Build history of the part. All positions in model axes, mm. Face numbers are marked on the shaded views. A direction names the side the tool comes from. Coordinates: 2 decimals unless noted, no trailing zeros. Order: outer loops, then holes, each group sorted by start corner. A loop starts at its lowest first (then second) coordinate and runs counter-clockwise, first axis right, second up. Notation, with made-up numbers: (19, 13) -> (77, 13) arc R10 ccw to (77, 26) -> close; hole circle Ø3 at (78.5, 35.5). An arc over 180 degrees is marked (long way). Write each question's results on one line, items separated by ' | '.
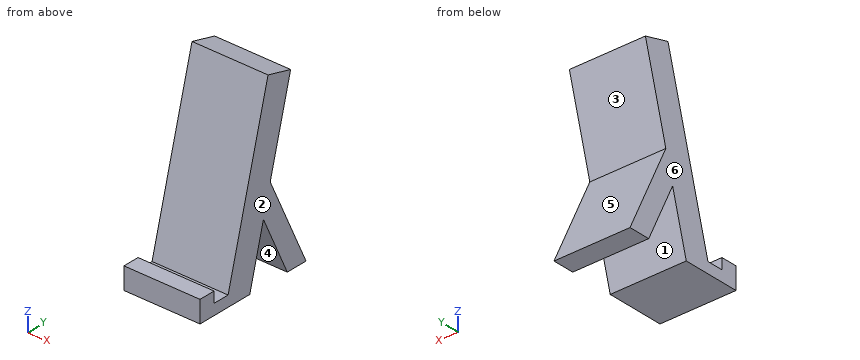
from build123d import *

# Parameters (mm, degrees)
F0_W     = 63.5
F0_H     = 25.4
F1_DEPTH = 19.05
F2_W     = 19.05
F2_H     = 12.7
F3_DEPTH = 63.5
F4_DEPTH = 25.4
F6_DEPTH = 88.9


with BuildPart() as f1:
    # F0 (on Front) → F1 (new body)
    with BuildSketch(Plane.XZ):
        with Locations((-31.75, 12.7)):
            Rectangle(F0_W, F0_H)
    extrude(amount=F1_DEPTH)

    # F2 (on Right) → F3 (join)
    with BuildSketch(Plane.YZ):
        with Locations((9.525, 6.35)):
            Rectangle(F2_W, F2_H)
        Polygon((19.05, 12.7), (19.05, 0), (48.5170639841, 0), (103.9536758859, 206.8922522169), (73.2855309012, 215.1097568989), align=None)
    extrude(amount=-F3_DEPTH)

    # F4 (add): a face of the model
    f4_faces = [f1.faces().sort_by_distance(p)[0] for p in [
        (0, 54.342102556, 96.7816110537),
    ]]
    extrude(f4_faces, amount=F4_DEPTH)

    # F5 (on face) → F6 (join)
    with BuildSketch(Plane.YZ.offset(25.4)):
        Polygon((124.8500692878, 0), (76.235369935, 103.4461261084), (67.012033734, 69.0241667908), (99.4500692878, 0), align=None)
    extrude(amount=-F6_DEPTH)


solid = f1.part
Item 1: Slice it at A-A, the plane x = -54.5. List the corners of the cut face in (y, z), and give its area (3 significant figures).
Answer:
outline: (-19.05, 0) -> (48.52, 0) -> (67.01, 69.02) -> (99.45, 0) -> (124.85, 0) -> (76.24, 103.45) -> (103.95, 206.89) -> (73.29, 215.11) -> (19.05, 12.7) -> (0, 12.7) -> (0, 25.4) -> (-19.05, 25.4) -> close | area: 9,830 mm^2
Item 2: Drill centre lines: line 1 (Z direction, x = 0, y = -6); line 2 (Y direction, x = 0.5, z = 12.5); line 3 (Z direction, x = 14, y = 15.5). Where is each one in solid material? Low to high. Write a range as from..to.
Answer:
line 1: z = 0..25.4 | line 2: y = -19.05..51.87, 93.58..118.98 | line 3: z = 0..12.7
Item 3: Pull direction Y, two halves, no side cores. Call the marked faces 1, 2, 3 and 4: released by +Y, released by -Y, zero draft, split by the parting line, or undercut.
Answer:
face 1: undercut | face 2: zero draft | face 3: released by +Y | face 4: undercut
Item 4: Slice it at B-B, the plane z = 65.5. List the corners of the cut face in (x, y), and give its area (3 significant figures).
Answer:
outline: (-63.5, 33.2) -> (25.4, 33.2) -> (25.4, 66.07) -> (-63.5, 66.07) -> close; (-63.5, 68.67) -> (25.4, 68.67) -> (25.4, 94.07) -> (-63.5, 94.07) -> close | area: 5,180 mm^2
Item 5: Pin check, flat tips, straight feed: pin 1 (5 mm diameter, centred on x = -26.5, z = 160.5, fed in from +Y); pin 2 (9.5 mm diameter, centred on x = -8, y = -11.5, fed in from +Z); pin 3 (2 mm diameter, centred on x = -2, z = 79, fed in from -Y). Stop position of each tip, or through.
Answer:
pin 1: stops at y = 92.19 | pin 2: stops at z = 25.4 | pin 3: stops at y = 36.55
Item 6: Slice it at C-C, the plane y = 13.5. List the corners of the cut face in (x, z), and give its area (3 significant figures).
Answer:
outline: (-63.5, 0) -> (25.4, 0) -> (25.4, 12.7) -> (-63.5, 12.7) -> close | area: 1,130 mm^2
Item 7: Slice it at D-D, the plane z = 144.5. List the corners of the cut face in (x, y), and give its area (3 significant figures).
Answer:
outline: (-63.5, 54.37) -> (25.4, 54.37) -> (25.4, 87.24) -> (-63.5, 87.24) -> close | area: 2,920 mm^2
Item 8: Tool access for the marked faces 5 and 6: list every direction of +Z, -Z, +X, -X, +Y, -Y with a clear straight run to the whole face (end or side of a thin tool).
Answer:
face 5: +X, -X, +Y | face 6: +Z, -Z, -X, +Y, -Y
